Design review of the part shown in the three views and the two pictorial views. Dimensions are in mm from the part's minimum x, y and z. A direction names the side the tool comes from. Give positions to 0.01 mm unless a question says otherwise; leave off trailing zeros. Loops run counter-clockwise (first coordinate to the right, second up) from the corner with the lowest first, then second, coordinate; pieces in that order, holes last. Notation, with made-up numbers: (15, 67.25) -> (71, 67.25) arc R22 cw to (71, 99.25) -> close; hole circle Ø3 at (33.25, -37.75). An arc over 180 degrees is marked (long way). Answer as CSV lines item,"result".
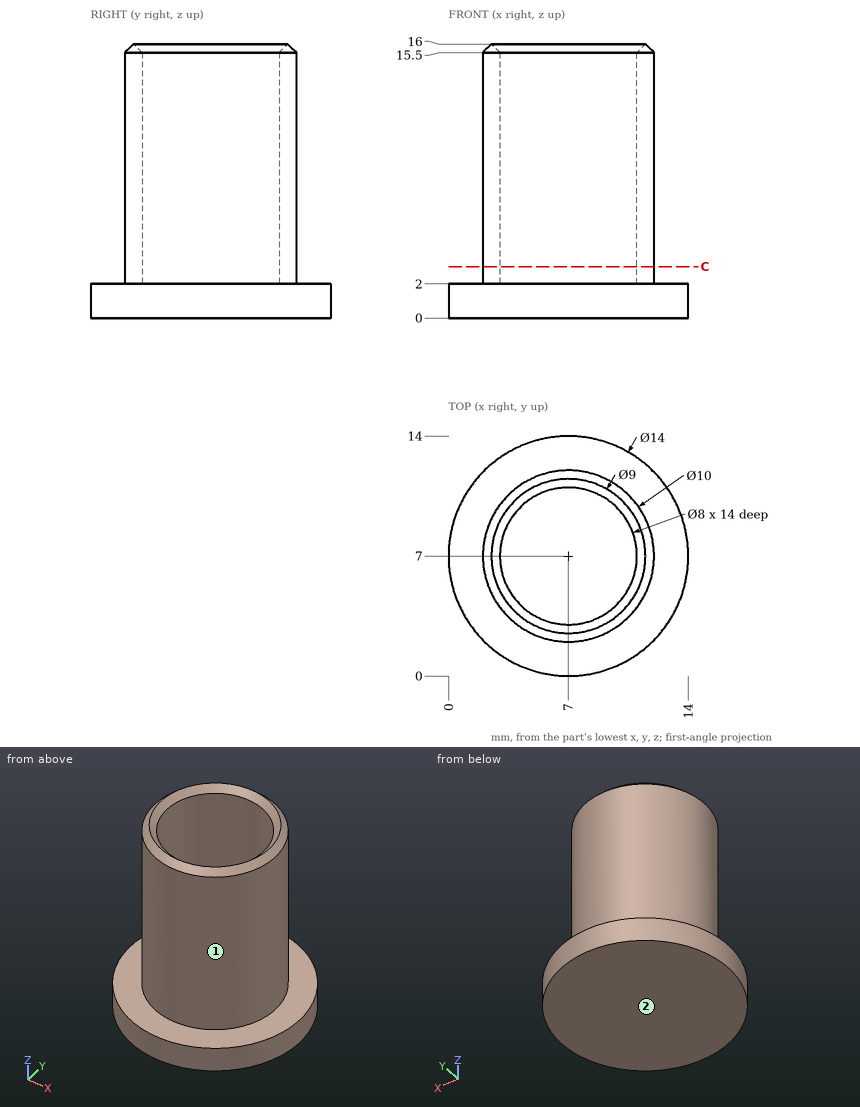
Q1. Clearance check with flat-ended pins moving along their axes: pin 1 Ø2 at (y, z) = (11.5, 5.5) entering from -X; pin 2 Ø4 at (x, y) = (7, 6) entering from +Z; pin 3 Ø4 at (x, z) = (5, 14) entering from +Y. State where each tip first meets the part, or that it passes through.
Filled sheet:
pin 1,"stops at x = 3.43"
pin 2,"stops at z = 2"
pin 3,"stops at y = 12"
Q2. We need section C-C, the plane z = 3. State the section outline as (x, y) points, and give its area (3 significant figures).
Filled sheet:
outline,"circle Ø10 at (7, 7); hole circle Ø8 at (7, 7)"
area,"28.3 mm^2"
Q3. For the marked faces 1 and 2, list the 3-axis set-ups (+Z, -Z, +X, -X, +Y, -Y) from which the entire face can be reached by the end or side of a thin tool; tool diameter is ignored.
Filled sheet:
face 1,"+Z"
face 2,"-Z, +X, -X, +Y, -Y"
Q4. To check wall thickness, follow probe 1 along Y at (x, z) = (7, 5); probe 2 along Z at (x, y) = (12.25, 10.5); probe 3 along Y at (x, z) = (10, 6.5). State the ranges of each line that lie inside material, in increasing order. Write a range as from..to.
Filled sheet:
probe 1,"y = 2..3, 11..12"
probe 2,"z = 0..2"
probe 3,"y = 3..4.35, 9.65..11"
